from build123d import *

# Parameters (mm, degrees)
F0_R     = 1.5
F1_DEPTH = 5
F2_R     = 2.5
F3_DEPTH = 1
F4_R     = 0.761295
F4_R_2   = 0.75
F5_DEPTH = 8


with BuildPart() as f1:
    # F0 (on Front) → F1 (new body)
    with BuildSketch(Plane.XZ):
        Circle(F0_R)
    extrude(amount=F1_DEPTH)

    # F2 (on face) → F3 (join)
    with BuildSketch(Plane.XZ.offset(5)):
        Circle(F2_R)
    extrude(amount=F3_DEPTH)

    # F4 (on face) → F5 (join)
    with BuildSketch(Plane.XZ.offset(6)):
        with Locations((0.984464, -1.048415)):
            Circle(F4_R)
        with Locations((-0.984464, -1.048415)):
            Circle(F4_R)
        with Locations((0, 0.944208)):
            Circle(F4_R_2)
    extrude(amount=F5_DEPTH)


solid = f1.part
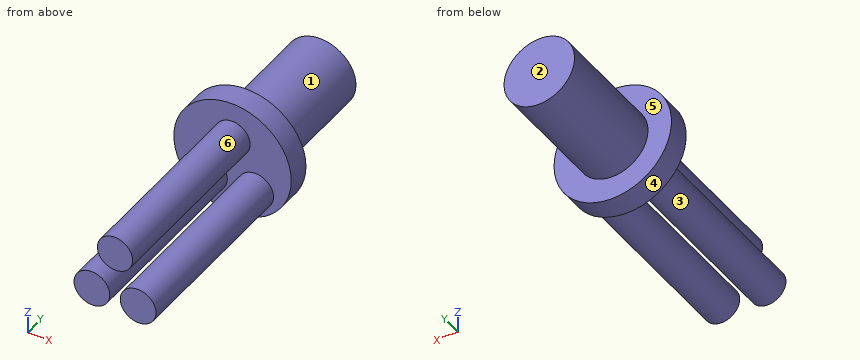
Read the model definition and answer for the solid it produces. Units are mm, in the model's axes. Face numbers are marked on the shaded views. A direction names the side the tool comes from. Round coordinates to 2 decimals unless told otherwise and drop trailing zeros. Order: outer loops, then holes, each group sorted by start corner. A loop starts at its lowest first (then second) coordinate and runs counter-clockwise, first axis right, second up.
1) The part is cut by section A-A on x = 0. Write down the section's boundary in (y, z), plus the area to 3 significant figures.
2) The mould has two halves that part along X. Classify the marked faces 1, 2 and 3: released by +X, released by -X, zero draft, split by the parting line, or undercut.
3) Flat-ended cylindrical pins translate along their axes: pin 1 (1 mm diameter, centred on x = -1.5, z = 0.5, fed in from -Y); pin 2 (1.5 mm diameter, centred on x = 2, y = -12, fed in from +Z). Find the tip coordinate at first contact, or state that the pin passes through.
4) Straight lines are drawn through the part: L1, parallel to Z at x = 1, y = -9.5; L2, parallel to Y at x = -1.3, z = -1.65; L3, parallel to Y at x = 0.4, z = -2.3. For each, find the intervals that lie inside material, in ascending order.
5) The part is cut by section C-C on y = -12. Write down the section's boundary in (x, z).
6) For the marked faces 4, 5 and 6, determine the directions among +Z, -Z, +X, -X, +Y, -Y from which every point of the face is accessible in a straight line to the end or side of a thin tool.
7) The part is cut by section B-B on z = 0. Write down the section's boundary in (x, y), plus the area to 3 significant figures.
8) The part is cut by section D-D on z = -0.55. Write down the section's boundary in (x, y), plus the area to 3 significant figures.
Resolved:
1. outline: (-14, 0.19) - (-6, 0.19) - (-6, -2.5) - (-5, -2.5) - (-5, -1.5) - (0, -1.5) - (0, 1.5) - (-5, 1.5) - (-5, 2.5) - (-6, 2.5) - (-6, 1.69) - (-14, 1.69) - close
1. area: 32.0 mm2
2. face 1: split by the parting line
2. face 2: zero draft
2. face 3: undercut
3. pin 1: stops at y = -6
3. pin 2: stops at z = -0.33
4. L1: z = -1.81 to -0.29
4. L2: y = -14 to -5
4. L3: y = -6 to -5
5. outline: circle Ø1.52 at (-0.98, -1.05); circle Ø1.5 at (0, 0.94); circle Ø1.52 at (0.98, -1.05)
6. face 4: +Y, -Y
6. face 5: +Y
6. face 6: -Y
7. outline: (-2.5, -6) - (2.5, -6) - (2.5, -5) - (1.5, -5) - (1.5, 0) - (-1.5, 0) - (-1.5, -5) - (-2.5, -5) - close
7. area: 20.0 mm2
8. outline: (-2.44, -6) - (-1.56, -6) - (-1.56, -14) - (-0.41, -14) - (-0.41, -6) - (0.41, -6) - (0.41, -14) - (1.56, -14) - (1.56, -6) - (2.44, -6) - (2.44, -5) - (1.4, -5) - (1.4, 0) - (-1.4, 0) - (-1.4, -5) - (-2.44, -5) - close
8. area: 37.2 mm2
